Source: CAD feature listing. Evaluate the final solid. Frame: model axes, mm. A direction names the side the tool comes from. Give positions to 0.01 mm unless a question says otherwise; leave off trailing zeros. Write each loop counter-clockwise with the first axis right and the second up, starting at its lowest first coordinate (ties: lowest second). Pieces come first, ordered by that corner, then holes. Notation, with made-up numbers: M 12,3.25 L 32,3.25 A26 ccw 32,29.25 Z; hole C 75,8 d7. An arc over 180 degrees is marked long. Return JSON: item names as keys, results as strings.
```python
from build123d import *

# Parameters (mm, degrees)
F0_R           = 5
F1_DEPTH       = 20
F3_D           = 6.3
F3_CBORE_D     = 11.25
F3_CBORE_DEPTH = 6
F4_SIZE        = 2.5


with BuildPart() as f1:
    # F0 (on Front) → F1 (new body)
    with BuildSketch(Plane.XZ):
        Polygon((-30, 16.25), (-30, -16.25), (30, -16.25), (30, 16.25), (17, 16.25), (17, 26.75), (-17, 26.75), (-17, 16.25), align=None)
        with Locations((0, 8.75)):
            Circle(F0_R, mode=Mode.SUBTRACT)
    extrude(amount=F1_DEPTH)

    # F3 (through all)
    with Locations(Plane.XY.offset(16.25)):
        with Locations((23, -10), (-23, -10)):
            CounterBoreHole(F3_D / 2, F3_CBORE_D / 2, F3_CBORE_DEPTH)

    # F4
    f4_edges = [f1.edges().sort_by_distance(p)[0] for p in [
        (17, -10, 26.75),
        (-17, -10, 26.75),
    ]]
    chamfer(f4_edges, length=F4_SIZE)


solid = f1.part
```
1) Contact query for flat-ended pins moving along their axis: pin 1 Ø5 at (x, y) = (-23, -10) entering from +Z; pin 2 Ø6.5 at (x, y) = (26.5, -13) entering from +Z; pin 3 Ø4 at (y, z) = (-6, 21.5) entering from +X; pin 4 Ø7 at (x, y) = (-23, -10) entering from +Z. Output: stop coordinate, or through.
Numbers:
{"pin 1": "passes through", "pin 2": "stops at z = 16.25", "pin 3": "stops at x = 17", "pin 4": "stops at z = 10.25"}
2) Cut plane A-A, the plane y = -10. Return the cut outline in (x, z) (3 decimals).
Numbers:
{"outline": "M -30,-16.25 L -26.15,-16.25 L -26.15,10.25 L -28.625,10.25 L -28.625,16.25 L -30,16.25 Z; M -19.85,-16.25 L 19.85,-16.25 L 19.85,10.25 L 17.375,10.25 L 17.375,16.25 L 17,16.25 L 17,24.25 L 14.5,26.75 L -14.5,26.75 L -17,24.25 L -17,16.25 L -17.375,16.25 L -17.375,10.25 L -19.85,10.25 Z; M 26.15,-16.25 L 30,-16.25 L 30,16.25 L 28.625,16.25 L 28.625,10.25 L 26.15,10.25 Z; hole C 0,8.75 d10"}
3) Cut plane B-B, the plane z = 8.75. Return the cut outline in (x, y).
Numbers:
{"outline": "M -30,-20 L -5,-20 L -5,0 L -30,0 Z; M 5,-20 L 30,-20 L 30,0 L 5,0 Z; hole C -23,-10 d6.3; hole C 23,-10 d6.3"}
4) Set-up query: faces 1 (the face through (26, -5, 16.25)), 2 (the face through (-20.6, -12.4, 10.25)), 3 (the face through (-26, -5, 16.25)). Return all of +Z, -Z, +X, -X, +Y, -Y with unobstructed straight access to the full face (end or side cutting, diameter ignored); none if empty.
Numbers:
{"face 1": "+Z, +X, +Y, -Y", "face 2": "+Z", "face 3": "+Z, -X, +Y, -Y"}
5) Line query: line 1 (Y direction, x = -23, z = -7.5); line 2 (Y direction, x = -23, z = 13.35) (3 decimals); line 3 (X direction, y = -14.5, z = 16) (3 decimals). Output: solid intervals per line, ascending. Write a range as [from, to].
Numbers:
{"line 1": "y = [-20, -13.15], [-6.85, 0]", "line 2": "y = [-20, -15.625], [-4.375, 0]", "line 3": "x = [-30, -26.375], [-19.625, 19.625], [26.375, 30]"}
6) Cut plane C-C, the plane x = 0. Return the cut outline in (y, z).
Numbers:
{"outline": "M -20,-16.25 L 0,-16.25 L 0,3.75 L -20,3.75 Z; M -20,13.75 L 0,13.75 L 0,26.75 L -20,26.75 Z"}
7) Cut plane D-D, the plane z = 3. Return the cut outline in (x, y).
Numbers:
{"outline": "M -30,-20 L 30,-20 L 30,0 L -30,0 Z; hole C -23,-10 d6.3; hole C 23,-10 d6.3"}
8) Draft query along Y for faces 4 (the face through (0, 0, 1)), 5 (the face through (30, -10, 0)), 6 (the face through (18.536, -13.423, 13.292)). Return one class per face: released by +Y, released by -Y, zero draft, split by the parting line, or undercut.
Numbers:
{"face 4": "released by +Y", "face 5": "zero draft", "face 6": "undercut"}
